from build123d import *

# Parameters (mm, degrees)
SKETCH010_W  = 20
SKETCH010_H  = 3
PAD008_DEPTH = 10
PAD009_DEPTH = 70
SKETCH012_W  = 20
SKETCH012_H  = 3
PAD010_DEPTH = 10
SKETCH014_W  = 20
SKETCH014_H  = 4
PAD012_DEPTH = 20
SKETCH018_R  = 9
POCKET_DEPTH = 1


with BuildPart() as part:
    # Sketch010 (on XY_Plane of Origin012) → Pad008 (new body)
    with BuildSketch(Plane.XY):
        Rectangle(SKETCH010_W, SKETCH010_H)
    extrude(amount=PAD008_DEPTH)

    # Sketch011 (on Face5 of Pad008) → Pad009 (join)
    with BuildSketch(Plane(origin=(0, 0, 0), x_dir=(1, 0, 0), z_dir=(0, 0, -1))):
        Polygon((-7.87868, 1.5), (-6.37868, 0), (-7.87868, -1.5), (-10, -1.5), (-10, 1.5), align=None)
        Polygon((7.87868, 1.5), (6.37868, 0), (7.87868, -1.5), (10, -1.5), (10, 1.5), align=None)
    extrude(amount=PAD009_DEPTH)

    # Sketch012 (on Face7 of Pad009) → Pad010 (join)
    with BuildSketch(Plane(origin=(0, 0, -70), x_dir=(1, 0, 0), z_dir=(0, 0, -1))):
        Rectangle(SKETCH012_W, SKETCH012_H)
    extrude(amount=PAD010_DEPTH)

    # Sketch014 (on Face10 of Pad010) → Pad012 (join)
    with BuildSketch(Plane.XZ.offset(1.5)):
        with Locations((0, 8)):
            Rectangle(SKETCH014_W, SKETCH014_H)
    extrude(amount=PAD012_DEPTH)

    # Sketch018 (on Face4 of Pad012) → Pocket (cut)
    with BuildSketch(Plane(origin=(0, 0, 6), x_dir=(1, 0, 0), z_dir=(0, 0, -1))):
        with Locations((0, 11.5)):
            Circle(SKETCH018_R)
    extrude(amount=-POCKET_DEPTH, mode=Mode.SUBTRACT)


solid = part.part
Geometry check sheet. Reference: the model listing, model coordinates, mm. A direction names the side the tool comes from. Give positions to 0.01 mm unless a question says otherwise; leave off trailing zeros. Order: outer loops, then holes, each group sorted by start corner. A loop starts at its lowest first (then second) coordinate and runs counter-clockwise, first axis right, second up.
1) Cross-section at B-B (x = 0). Record the boundary of the cut face in (y, z), then the cut area to 3 significant figures.
Results are:
outline: (-21.5, 6) - (-20.5, 6) - (-20.5, 7) - (-2.5, 7) - (-2.5, 6) - (-1.5, 6) - (-1.5, 0) - (1.5, 0) - (1.5, 10) - (-21.5, 10) - close; (-1.5, -80) - (1.5, -80) - (1.5, -70) - (-1.5, -70) - close
area: 122 mm2
2) Cross-section at A-A (z = -45). Record the boundary of the cut face in (x, y), then the cut area to 3 significant figures.
Results are:
outline: (-10, -1.5) - (-7.88, -1.5) - (-6.38, 0) - (-7.88, 1.5) - (-10, 1.5) - close; (6.38, 0) - (7.88, -1.5) - (10, -1.5) - (10, 1.5) - (7.88, 1.5) - close
area: 17.2 mm2
3) Draft check along Y on faces 4 (the flat face through (7.14, -0.76, -34.51)), 5 (the cylindrical face through (-1.951, -2.714, 6.493)), 6 (the flat face through (0, 0, -70)). Enter one of: released by +Y, released by -Y, zero draft, split by the parting line, or undercut.
Results are:
face 4: released by -Y
face 5: undercut
face 6: zero draft
4) Gauge pin test, flat end, axial feed: pin 1 (1 mm diameter, centred on x = -5, z = -12.5, fed in from -Y). Record the tip position at first contact, or that the pin passes through.
Results are:
pin 1: passes through
5) Cross-section at D-D (x = 5.25). Record the boundary of the cut face in (y, z), then the cut area to 3 significant figures.
Results are:
outline: (-21.5, 6) - (-18.81, 6) - (-18.81, 7) - (-4.19, 7) - (-4.19, 6) - (-1.5, 6) - (-1.5, 0) - (1.5, 0) - (1.5, 10) - (-21.5, 10) - close; (-1.5, -80) - (1.5, -80) - (1.5, -70) - (-1.5, -70) - close
area: 125 mm2
6) Cross-section at C-C (y = -11.5). Record the boundary of the cut face in (x, z).
Results are:
outline: (-10, 6) - (-9, 6) - (-9, 7) - (9, 7) - (9, 6) - (10, 6) - (10, 10) - (-10, 10) - close
7) Tool access check on faces 1 (the flat face through (0, -12, 7)), 2 (the flat face through (-7.14, -0.76, -34.51)), 3 (the flat face through (7.12, 0.74, -34.51)). Record the directions out of +Z, -Z, +X, -X, +Y, -Y that give a thin tool (end or side, any length) a straight path to the whole face; none if there is none.
Results are:
face 1: -Z
face 2: -Y
face 3: +Y
8) Material ranges on probe 1 along Y at (x, z) = (0, 6.65); probe 2 along X at (y, z) = (-11.5, 6.45); probe 3 along Z at (x, y) = (2.25, -12.5), recorded low to high.
Results are:
probe 1: y = -21.5 to -20.5, -2.5 to 1.5
probe 2: x = -10 to -9, 9 to 10
probe 3: z = 7 to 10
